```python
from build123d import *

# Parameters (mm, degrees)
BASE_FLANGE1_DEPTH   = 0.7366
FILLET1_R            = 5
FILLET2_R            = 5
FILLET3_R            = 5
FILLET4_R            = 5
EDGE_FLANGE2_START   = -47.5
EDGE_FLANGE2_DEPTH   = 15.3683
EDGE_FLANGE2_START_2 = -32.5
EDGE_FLANGE2_2_DEPTH = 0.3683
EDGE_FLANGE2_3_DEPTH = 15
FILLET7_R            = 5
FILLET8_R            = 5
SKETCH18_R           = 1.5
CUT_EXTRUDE1_DEPTH   = 40
SKETCH23_R           = 1.52
CUT_EXTRUDE6_DEPTH   = 30
SKETCH25_R           = 1.4
CUT_EXTRUDE8_DEPTH   = 10


with BuildPart() as part:
    # Base-Flange1: sheet metal written as solids
    # Sketch1 → Base-Flange1 (new body)
    with BuildSketch(Plane(origin=(0, 0, 0), x_dir=(1, 0, 0), z_dir=(0, 1, 0))):
        Polygon((19.610938441, 32.5), (65, 32.5), (65, -32.5), (-65, -32.5), (-65, 32.5), (-19.610938441, 32.5), (-11.999061559, 32.5), (-11.999061559, 47.5), (12.000938441, 47.5), (12.000938441, 32.5), align=None)
    extrude(amount=-BASE_FLANGE1_DEPTH)

    # Fillet1
    fillet1_edges = [part.edges().sort_by_distance(p)[0] for p in [
        (65, -0.3683, 32.5),
    ]]
    fillet(fillet1_edges, radius=FILLET1_R)

    # Fillet2
    fillet2_edges = [part.edges().sort_by_distance(p)[0] for p in [
        (65, -0.3683, -32.5),
    ]]
    fillet(fillet2_edges, radius=FILLET2_R)

    # Fillet3
    fillet3_edges = [part.edges().sort_by_distance(p)[0] for p in [
        (-65, -0.3683, 32.5),
    ]]
    fillet(fillet3_edges, radius=FILLET3_R)

    # Fillet4
    fillet4_edges = [part.edges().sort_by_distance(p)[0] for p in [
        (-65, -0.3683, -32.5),
    ]]
    fillet(fillet4_edges, radius=FILLET4_R)

    # Edge-Flange2: read off the stored shape, not the designer's step
    # Edge-Flange2 outline → Edge-Flange2 (cut)
    with BuildSketch(Plane.XY.offset(EDGE_FLANGE2_START)):
        with BuildLine():
            ThreePointArc((-11.999061559, -0.197371375), (-11.643753776, -0.050198073), (-11.262461559, 0))
            Line((-11.262461559, 0), (-11.999061559, 0))
            Line((-11.999061559, 0), (-11.999061559, -0.197371375))
        make_face()
        with BuildLine():
            ThreePointArc((11.264338441, 0), (11.645630659, -0.050198073), (12.000938441, -0.197371375))
            Line((12.000938441, -0.197371375), (12.000938441, 0))
            Line((12.000938441, 0), (11.264338441, 0))
        make_face()
    extrude(amount=EDGE_FLANGE2_DEPTH, mode=Mode.SUBTRACT)

    # Edge-Flange2 2 outline → Edge-Flange2 2 (cut)
    with BuildSketch(Plane.XY.offset(EDGE_FLANGE2_START_2)):
        with BuildLine():
            Line((-11.999061559, -0.7366), (-10.894161559, -0.7366))
            Line((-10.894161559, -0.7366), (-10.894161559, 0))
            Line((-10.894161559, 0), (-11.262461559, 0))
            ThreePointArc((-11.262461559, 0), (-11.643753776, -0.050198073), (-11.999061559, -0.197371375))
            Line((-11.999061559, -0.197371375), (-11.999061559, -0.7366))
        make_face()
        with BuildLine():
            Line((12.000938441, -0.7366), (12.000938441, -0.197371375))
            ThreePointArc((12.000938441, -0.197371375), (11.645630659, -0.050198073), (11.264338441, 0))
            Line((11.264338441, 0), (10.896038441, 0))
            Line((10.896038441, 0), (10.896038441, -0.7366))
            Line((10.896038441, -0.7366), (12.000938441, -0.7366))
        make_face()
    extrude(amount=EDGE_FLANGE2_2_DEPTH, mode=Mode.SUBTRACT)

    # Edge-Flange2 3 outline → Edge-Flange2 3 (add)
    with BuildSketch(Plane.XY.offset(EDGE_FLANGE2_START)):
        with BuildLine():
            ThreePointArc((-11.999061559, -1.4732), (-11.783316414, -0.952345145), (-11.262461559, -0.7366))
            Line((-11.262461559, -0.7366), (-11.999061559, -0.7366))
            Line((-11.999061559, -0.7366), (-11.999061559, -0.197371375))
            ThreePointArc((-11.999061559, -0.197371375), (-12.538290183, -0.7366), (-12.735661559, -1.4732))
            Line((-12.735661559, -1.4732), (-12.735661559, -15))
            Line((-12.735661559, -15), (-11.999061559, -15))
            Line((-11.999061559, -15), (-11.999061559, -1.4732))
        make_face()
        with BuildLine():
            Line((12.737538441, -15), (12.737538441, -1.4732))
            ThreePointArc((12.737538441, -1.4732), (12.540167066, -0.7366), (12.000938441, -0.197371375))
            Line((12.000938441, -0.197371375), (12.000938441, -0.7366))
            Line((12.000938441, -0.7366), (11.264338441, -0.7366))
            ThreePointArc((11.264338441, -0.7366), (11.785193296, -0.952345145), (12.000938441, -1.4732))
            Line((12.000938441, -1.4732), (12.000938441, -15))
            Line((12.000938441, -15), (12.737538441, -15))
        make_face()
    extrude(amount=EDGE_FLANGE2_3_DEPTH)

    # Fillet7
    fillet7_edges = [part.edges().sort_by_distance(p)[0] for p in [
        (12.369238441, -15, -47.5),
    ]]
    fillet(fillet7_edges, radius=FILLET7_R)

    # Fillet8
    fillet8_edges = [part.edges().sort_by_distance(p)[0] for p in [
        (-12.367361559, -15, -47.5),
    ]]
    fillet(fillet8_edges, radius=FILLET8_R)

    # Sketch18 → Cut-Extrude1 (cut)
    with BuildSketch(Plane.ZY.offset(12.735661559)):
        with Locations(Location((-39.810498868, -4.68598948, 0), (0, 0, 270))):
            Circle(SKETCH18_R)
        with BuildLine():
            ThreePointArc((-39.496869826, -12.179429066), (-38.060907717, -10.61801534), (-39.622321443, -9.182053232))
            ThreePointArc((-39.622321443, -9.182053232), (-42.925238149, -7.933819403), (-44.310498868, -4.68598948))
            ThreePointArc((-44.310498868, -4.68598948), (-45.810498868, -3.18598948), (-47.310498868, -4.68598948))
            ThreePointArc((-47.310498868, -4.68598948), (-45.001731004, -10.099039351), (-39.496869826, -12.179429066))
        make_face()
    extrude(amount=-CUT_EXTRUDE1_DEPTH, mode=Mode.SUBTRACT)

    # Sketch23 → Cut-Extrude6 (cut)
    with BuildSketch(Plane(origin=(13.900294902, -27.805223525, -244.007014279), x_dir=(-3.6601011800335994e-15, 0.31934249234828205, -0.9476393684207024), z_dir=(1, 0, 0))):
        with Locations(Location((-186.121703077, 87.117320509, 0), (0, 0, 251.376833723))):
            Circle(SKETCH23_R)
    extrude(amount=-CUT_EXTRUDE6_DEPTH, mode=Mode.SUBTRACT)

    # Sketch25 → Cut-Extrude8 (cut)
    with BuildSketch(Plane(origin=(-71.983966672, 0, -96.098250098), x_dir=(1, 0, 0), z_dir=(0, 1, 0))):
        with Locations(Location((79.090906604, -126.157708005, 0), (0, 0, 270))):
            Circle(SKETCH25_R)
        with Locations(Location((69.540906604, -126.157708005, 0), (0, 0, 270))):
            Circle(SKETCH25_R)
    extrude(amount=-CUT_EXTRUDE8_DEPTH, mode=Mode.SUBTRACT)


solid = part.part
```
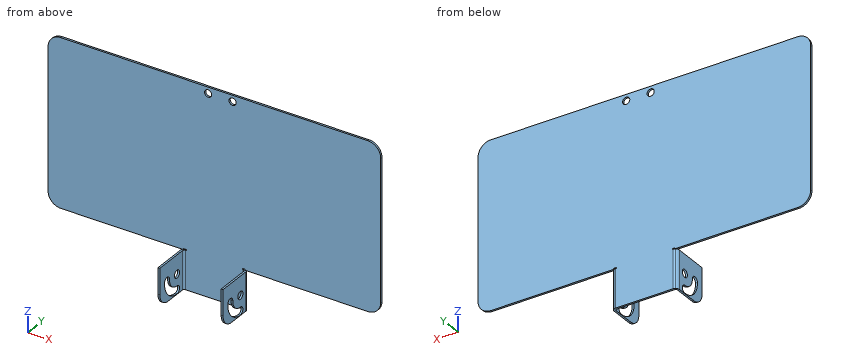
Design review of the part built by this model. Coordinates are the model's own, in mm. Give positions to 0.01 mm unless a question says otherwise; leave off trailing zeros. Write each loop counter-clockwise with the first axis right and the second up, starting at its lowest first coordinate (ties: lowest second). Pieces come first, ordered by that corner, then holes. Notation, with made-up numbers: (6, -2) -> (22, -2) arc R25 ccw to (22, 36) -> close; hole circle Ø4 at (20, 28). An arc over 180 degrees is marked (long way). Answer in a Markdown table with one row per item.
(1) Consider section B-B (x = 22). State the section outline as (y, z) points, then the cut area to 3 significant figures.
Results:
| item | result |
|---|---|
| outline | (-0.74, -32.5) -> (0, -32.5) -> (0, 32.5) -> (-0.74, 32.5) -> close |
| area | 47.9 mm2 |
(2) Consider section A-A (z = -25). State the section outline as (x, y) points.
Results:
| item | result |
|---|---|
| outline | (-65, -0.74) -> (65, -0.74) -> (65, 0) -> (-65, 0) -> close |
(3) To check wall thickness, follow probe 1 along X at (y, z) = (-5.25, -42); probe 2 along Y at (x, z) = (-29, -24). State the ranges of each line that lie inside material, in increasing order.
Results:
| item | result |
|---|---|
| probe 1 | -12.74 to -12, 12 to 12.74 |
| probe 2 | -0.74 to 0 |
(4) Clearance check with flat-ended pins moving along their axes: pin 1 (0.6 mm diameter, centred on x = -30, y = -0.5, fed in from -Z); pin 2 (7 mm diameter, centred on y = -10, z = -37, fed in from +X); pin 3 (6 mm diameter, centred on y = -6, z = -23, fed in from -X); pin 4 (3.5 mm diameter, centred on y = -4.69, z = -39.81, fed in from -X). State where each tip first meets the part, or that it passes through.
Results:
| item | result |
|---|---|
| pin 1 | z = -32.5 |
| pin 2 | x = 12.74 |
| pin 3 | through |
| pin 4 | x = -12.74 |
